```python
from build123d import *

# Parameters (mm, degrees)
F1_DEPTH = 304.8
F2_R     = 15.24
F3_DEPTH = 81.546806
F4_W     = 35.56
F4_H     = 6.35
F5_DEPTH = 81.546806


with BuildPart() as f1:
    # F0 (on Right) → F1 (new body)
    with BuildSketch(Plane.YZ):
        Polygon((0, 81.545806), (0, 0), (76.2, 0), (76.2, 50.8), (74.877944, 51.333434), align=None)
        Polygon((76.2, 54.61), (74.877944, 51.333434), (76.2, 50.8), align=None)
    extrude(amount=-F1_DEPTH)

    # F2 (on Top) → F3 (cut, through all)
    with BuildSketch(Plane.XY):
        with Locations((-156.039268, 38.1)):
            Circle(F2_R)
    extrude(amount=F3_DEPTH, mode=Mode.SUBTRACT)

    # F4 (on face) → F5 (cut, through all)
    with BuildSketch(Plane(origin=(0, 0, 0), x_dir=(1, 0, 0), z_dir=(0, 0, -1))):
        with Locations((-156.136081, -38.1)):
            Rectangle(F4_W, F4_H)
    extrude(amount=-F5_DEPTH, mode=Mode.SUBTRACT)


solid = f1.part
```
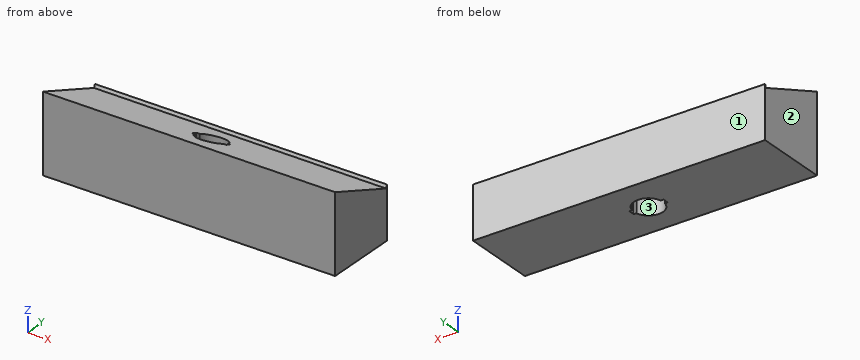
Could you check a few things on this model? Use its own coordinates, in mm. Face numbers are marked on the shaded views. Give positions to 0.01 mm unless a question says otherwise; leave off trailing zeros. Write each loop counter-clockwise with the first axis right and the second up, starting at its lowest first coordinate (ties: lowest second). Pieces come first, ordered by that corner, then holes. Notation, with made-up numbers: (67, 37.25) - (75, 37.25) arc R35 cw to (75, 71.25) - close; hole circle Ø8 at (32.25, 60.25). An arc over 180 degrees is marked (long way). One line per item, written item: value. Start each with the question number.
Item 1: If we mould it in two halves opening along Y, with no side actions, what happens to the marked faces 1, 2 and 3? For each: +Y half, -Y half, draft (parallel to the pull), parting line (faces both ways), or undercut.
Item 2: Imagine slicing it at D-D, the plane y = 31. List the corners of the cut face in (x, z) for me, and give its area (3 significant figures).
Item 3: Imagine slicing it at C-C, the plane x = -119. List the corners of the cut face in (y, z) for me.
Item 4: Imagine slicing it at B-B, the plane y = 48. List the corners of the cut face in (x, z) for me, and give its area (3 significant figures).
Item 5: I'm going to push flat-ended pins straight in: pin 1 (2 mm diameter, centred on x = -84.5, y = 14, fed in from +Z); pin 2 (6 mm diameter, centred on x = -151, y = 67.5, fed in from +Z). Where does each tip first touch, or does it pass through?
Item 6: Please list where these lines run through material, in increasing order: line 1 (X direction, y = 38.5, z = 29); line 2 (Y direction, x = -169, z = 14); line 3 (X direction, y = 33.5, z = 26.5). Write a range as from..to.
Item 7: Imagine slicing it at A-A, the plane z = 31. List the corners of the cut face in (x, y) for me (3 decimals).
Geometry says:
1. face 1: +Y half
1. face 2: draft
1. face 3: undercut
2. outline: (-304.8, 0) - (-169.52, 0) - (-169.52, 69.04) - (-304.8, 69.04) - close; (-142.55, 0) - (0, 0) - (0, 69.04) - (-142.55, 69.04) - close
2. area: 19,200 mm^2
3. outline: (0, 0) - (76.2, 0) - (76.2, 54.61) - (74.88, 51.33) - (0, 81.55) - close
4. outline: (-304.8, 0) - (-167.63, 0) - (-167.63, 62.18) - (-304.8, 62.18) - close; (-144.45, 0) - (0, 0) - (0, 62.18) - (-144.45, 62.18) - close
4. area: 17,500 mm^2
5. pin 1: z = 76.3
5. pin 2: z = 55.52
6. line 1: -304.8..-173.92, -138.36..0
6. line 2: 0..30.08, 46.12..76.2
6. line 3: -304.8..-170.57, -141.51..0
7. outline: (-304.8, 0) - (0, 0) - (0, 76.2) - (-304.8, 76.2) - close; hole (-173.916, 34.925) - (-170.945, 34.925) arc R15.24 ccw to (-141.134, 34.925) - (-138.356, 34.925) - (-138.356, 41.275) - (-141.134, 41.275) arc R15.24 ccw to (-170.945, 41.275) - (-173.916, 41.275) - close
